```python
from build123d import *

# Parameters (mm, degrees)
F0_R     = 158.75
F1_DEPTH = 23.495
F3_R     = 110.49
F3_R_2   = 29
F4_DEPTH = 7.5
F5_DEPTH = 11.945


# Not quite as in the source:
# - a fillet or chamfer that OpenCascade refuses, or shapes differently, is made with other operations: its cross-section is extruded or revolved along the edge and cut away or added


with BuildPart() as f1:
    # F0 (on Front) → F1 (new body)
    with BuildSketch(Plane.XZ):
        Circle(F0_R)
    extrude(amount=F1_DEPTH)

    # F2: fillet of radius 25 on 1 edges, made by hand

    # F2_s1 → F2_t2 (revolve, cut)
    with BuildSketch(Plane.XY):
        with BuildLine():
            ThreePointArc((158.75, -23.495), (150.9326547089, -6.7980083507), (133.7953416172, 0))
            Line((133.7953416172, 0), (158.75, 0))
            Line((158.75, 0), (158.75, -23.495))
        make_face()
    revolve(axis=Axis((0, 0, 0), (0, -1, 0)), mode=Mode.SUBTRACT)

    # F3 (on face) → F4 (cut)
    with BuildSketch(Plane(origin=(0, 0, 0), x_dir=(-1, 0, 0), z_dir=(0, 1, 0))):
        Circle(F3_R)
        Circle(F3_R_2, mode=Mode.SUBTRACT)
    extrude(amount=-F4_DEPTH, mode=Mode.SUBTRACT)

    # F5 (add): a face of the model
    f5_faces = [f1.faces().sort_by_distance(p)[0] for p in [
        (0, 0, 0),
    ]]
    extrude(f5_faces, amount=F5_DEPTH)

    # F6: F1 across face


with BuildPart() as f1_1:
    add(f1.part)
    add(f1.part.mirror(Plane.XZ.offset(23.495)))


solid = f1_1.part
```
Can you work these out from the model? Positions are in its coordinate system, mm. A direction names the side the tool comes from. Give positions to 0.01 mm unless a question says otherwise; leave off trailing zeros. Loops run counter-clockwise (first coordinate to the right, second up) from the corner with the lowest first, then second, coordinate; pieces in that order, holes last. Notation, with made-up numbers: M 63,-34.75 L 89,-34.75 A20 cw 89,-18.75 Z; hole C 35,0 d3. An arc over 180 degrees is marked long. One line per question, with ' | ' between items. Start each with the question number.
Q1. For faces 1 (the flat face through (-23, -7.5, -23)), 2 (the flat face through (0, -58.935, 0)), 3 (the cylindrical face through (23.952, -43.293, -107.863)), which set-ups out of +Z, -Z, +X, -X, +Y, -Y let a thin tool reach every point of the face, with its end or its side?
Q2. If we section it at C-C (y = -34.5): Please give me the cut outline in (x, z), plus the area to 3 significant figures.
Q3. If we section it at A-A (z = 0): Please give me the cut outline in (x, y) (3 decimals).
Q4. If we mould it in two halves opening along Z, with no side actions, what happens to faces 4 (the cylindrical face through (-13.38, -49.08, -25.73)), 5 (the flat face through (19, -46.99, 110))? For each: +Z half, -Z half, draft (parallel to the pull), parting line (faces both ways), or undercut.
Q5. If we section it at B-B (x = 0): Please give me the cut outline in (y, z) (3 decimals).
Q6. If I drill on line 1 (Z direction, x = 0, y = -41.5); line 2 (Z direction, x = 0, y = -5); line 3 (Z direction, x = -1, y = -55), over which ranges is the centre line in solid material (lowest first)? Write a range as from..to.
Q7. For pin 1 Ø5 at (x, z) = (124, -28.5) entering from -Y; pin 2 Ø4 at (x, z) = (38.5, 47.5) entering from +Y; pin 3 Ø1 at (x, y) = (-4, -36.5) entering from -Z, each with a flat end and sliding along its axis, tell me the tip position at first contact or that it passes through.
Computed:
1) face 1: +Y | face 2: +Z, -Z, +X, -X, -Y | face 3: -Y
2) outline: C 0,0 d310.88 | area: 75,900 mm²
3) outline: M -158.75,-23.495 A25 ccw -133.795,-46.99 L -110.49,-46.99 L -110.49,-39.49 L -29,-39.49 L -29,-58.935 L 29,-58.935 L 29,-39.49 L 110.49,-39.49 L 110.49,-46.99 L 133.795,-46.99 A25 ccw 158.75,-23.495 A25 ccw 133.795,0 L 110.49,0 L 110.49,-7.5 L 29,-7.5 L 29,11.945 L -29,11.945 L -29,-7.5 L -110.49,-7.5 L -110.49,0 L -133.795,0 A25 ccw Z
4) face 4: undercut | face 5: draft
5) outline: M -58.935,-29 L -39.49,-29 L -39.49,-110.49 L -46.99,-110.49 L -46.99,-133.795 A25 ccw -23.495,-158.75 A25 ccw 0,-133.795 L 0,-110.49 L -7.5,-110.49 L -7.5,-29 L 11.945,-29 L 11.945,29 L -7.5,29 L -7.5,110.49 L 0,110.49 L 0,133.795 A25 ccw -23.495,158.75 A25 ccw -46.99,133.795 L -46.99,110.49 L -39.49,110.49 L -39.49,29 L -58.935,29 Z
6) line 1: z = -149.43..-110.49, -29..29, 110.49..149.43 | line 2: z = -148.8..-110.49, -29..29, 110.49..148.8 | line 3: z = -28.98..28.98
7) pin 1: stops at y = -46.99 | pin 2: stops at y = -7.5 | pin 3: stops at z = -154.45
